from build123d import *

# Parameters (mm, degrees)
SKETCH_1_W          = 60
SKETCH_1_H          = 17
EXTRUDE_1_DEPTH     = 1.2
CUT_EXTRUDE_1_REACH = 33.204
SKETCH_4_R          = 3.25
SKETCH_4_W          = 9.6
SKETCH_4_H          = 3.4
SKETCH_4_W_2        = 7
SKETCH_4_H_2        = 3.5
SKETCH_4_W_3        = 8
SKETCH_4_H_3        = 2.9
SKETCH_4_W_4        = 8.4
SKETCH_4_H_4        = 3.2
SKETCH_4_W_5        = 6.5
FILLET_2_R          = 1
CHAMFER_1_SIZE      = 0.6
SKETCH_5_W          = 1.5
SKETCH_5_H          = 8
EXTRUDE_2_DEPTH     = 1.2
SKETCH_6_W          = 28.5
SKETCH_6_H          = 1.6
EXTRUDE_3_DEPTH     = 4
FILLET_3_R          = 1
CHAMFER_2_SIZE      = 1
CHAMFER_4_SIZE      = 1
FILLET_4_R          = 2
CHAMFER_5_SIZE      = 0.4


with BuildPart() as part:
    # 草图1 → 凸台-拉伸1 (new body)
    with BuildSketch(Plane(origin=(0, 0, 0), x_dir=(1, 0, 0), z_dir=(0, 1, 0))):
        Rectangle(SKETCH_1_W, SKETCH_1_H)
    extrude(amount=EXTRUDE_1_DEPTH)

    # 草图4 → 切除-拉伸1 (cut, up to next)
    with BuildSketch(Plane(origin=(0, 1.2, 0), x_dir=(1, 0, 0), z_dir=(0, 1, 0)), mode=Mode.PRIVATE) as cut_extrude_1_sk1:
        with Locations(Location((22.298485985, 3.98318929, 0), (0, 0, 270))):
            Circle(SKETCH_4_R)
    cut_extrude_1_tool1 = extrude(cut_extrude_1_sk1.sketch, amount=-CUT_EXTRUDE_1_REACH, mode=Mode.PRIVATE) & part.part
    # 草图4 → 切除-拉伸1 (cut, up to next)
    with BuildSketch(Plane(origin=(0, 1.2, 0), x_dir=(1, 0, 0), z_dir=(0, 1, 0)), mode=Mode.PRIVATE) as cut_extrude_1_sk2:
        with Locations((-20.471722325, 2.6)):
            Rectangle(SKETCH_4_W, SKETCH_4_H)
    cut_extrude_1_tool2 = extrude(cut_extrude_1_sk2.sketch, amount=-CUT_EXTRUDE_1_REACH, mode=Mode.PRIVATE) & part.part
    # 草图4 → 切除-拉伸1 (cut, up to next)
    with BuildSketch(Plane(origin=(0, 1.2, 0), x_dir=(1, 0, 0), z_dir=(0, 1, 0)), mode=Mode.PRIVATE) as cut_extrude_1_sk3:
        with Locations((-5.682926277, 2.55)):
            Rectangle(SKETCH_4_W_2, SKETCH_4_H_2)
    cut_extrude_1_tool3 = extrude(cut_extrude_1_sk3.sketch, amount=-CUT_EXTRUDE_1_REACH, mode=Mode.PRIVATE) & part.part
    # 草图4 → 切除-拉伸1 (cut, up to next)
    with BuildSketch(Plane(origin=(0, 1.2, 0), x_dir=(1, 0, 0), z_dir=(0, 1, 0)), mode=Mode.PRIVATE) as cut_extrude_1_sk4:
        with Locations((7.788485985, 2.55)):
            Rectangle(SKETCH_4_W_2, SKETCH_4_H_2)
    cut_extrude_1_tool4 = extrude(cut_extrude_1_sk4.sketch, amount=-CUT_EXTRUDE_1_REACH, mode=Mode.PRIVATE) & part.part
    # 草图4 → 切除-拉伸1 (cut, up to next)
    with BuildSketch(Plane(origin=(0, 1.2, 0), x_dir=(1, 0, 0), z_dir=(0, 1, 0)), mode=Mode.PRIVATE) as cut_extrude_1_sk5:
        with Locations((21.05, -4.584803861)):
            Rectangle(SKETCH_4_W_3, SKETCH_4_H_3)
    cut_extrude_1_tool5 = extrude(cut_extrude_1_sk5.sketch, amount=-CUT_EXTRUDE_1_REACH, mode=Mode.PRIVATE) & part.part
    # 草图4 → 切除-拉伸1 (cut, up to next)
    with BuildSketch(Plane(origin=(0, 1.2, 0), x_dir=(1, 0, 0), z_dir=(0, 1, 0)), mode=Mode.PRIVATE) as cut_extrude_1_sk6:
        with Locations((7.4, -4.734803861)):
            Rectangle(SKETCH_4_W_4, SKETCH_4_H_4)
    cut_extrude_1_tool6 = extrude(cut_extrude_1_sk6.sketch, amount=-CUT_EXTRUDE_1_REACH, mode=Mode.PRIVATE) & part.part
    # 草图4 → 切除-拉伸1 (cut, up to next)
    with BuildSketch(Plane(origin=(0, 1.2, 0), x_dir=(1, 0, 0), z_dir=(0, 1, 0)), mode=Mode.PRIVATE) as cut_extrude_1_sk7:
        with Locations((-7.25, -4.884803861)):
            Rectangle(SKETCH_4_W_5, SKETCH_4_H_2)
    cut_extrude_1_tool7 = extrude(cut_extrude_1_sk7.sketch, amount=-CUT_EXTRUDE_1_REACH, mode=Mode.PRIVATE) & part.part
    # 草图4 → 切除-拉伸1 (cut, up to next)
    with BuildSketch(Plane(origin=(0, 1.2, 0), x_dir=(1, 0, 0), z_dir=(0, 1, 0)), mode=Mode.PRIVATE) as cut_extrude_1_sk8:
        with Locations((-20.471722325, -4.834803861)):
            Rectangle(SKETCH_4_W, SKETCH_4_H)
    cut_extrude_1_tool8 = extrude(cut_extrude_1_sk8.sketch, amount=-CUT_EXTRUDE_1_REACH, mode=Mode.PRIVATE) & part.part
    add(cut_extrude_1_tool1.solids().sort_by_distance((22.298486, 1.2, -3.983189))[0], mode=Mode.SUBTRACT)
    add(cut_extrude_1_tool2.solids().sort_by_distance((-20.471722, 1.2, -2.6))[0], mode=Mode.SUBTRACT)
    add(cut_extrude_1_tool3.solids().sort_by_distance((-5.682926, 1.2, -2.55))[0], mode=Mode.SUBTRACT)
    add(cut_extrude_1_tool4.solids().sort_by_distance((7.788486, 1.2, -2.55))[0], mode=Mode.SUBTRACT)
    add(cut_extrude_1_tool5.solids().sort_by_distance((21.05, 1.2, 4.584804))[0], mode=Mode.SUBTRACT)
    add(cut_extrude_1_tool6.solids().sort_by_distance((7.4, 1.2, 4.734804))[0], mode=Mode.SUBTRACT)
    add(cut_extrude_1_tool7.solids().sort_by_distance((-7.25, 1.2, 4.884804))[0], mode=Mode.SUBTRACT)
    add(cut_extrude_1_tool8.solids().sort_by_distance((-20.471722, 1.2, 4.834804))[0], mode=Mode.SUBTRACT)

    # 圆角2
    fillet_2_edges = [part.edges().sort_by_distance(p)[0] for p in [
        (-9.182926277, 0.6, -4.3),
        (-2.182926277, 0.6, -4.3),
        (4.288485985, 0.6, -4.3),
        (11.288485985, 0.6, -4.3),
        (17.05, 0.6, 6.034803861),
        (25.05, 0.6, 6.034803861),
        (3.2, 0.6, 6.334803861),
        (3.2, 0.6, 3.134803861),
        (11.6, 0.6, 3.134803861),
        (11.6, 0.6, 6.334803861),
        (-10.5, 0.6, 6.634803861),
        (-10.5, 0.6, 3.134803861),
        (-4, 0.6, 3.134803861),
        (-4, 0.6, 6.634803861),
        (-25.271722325, 0.6, 6.534803861),
        (-25.271722325, 0.6, 3.134803861),
        (-15.671722325, 0.6, 3.134803861),
        (-15.671722325, 0.6, 6.534803861),
        (-25.271722325, 0.6, -0.9),
        (-25.271722325, 0.6, -4.3),
        (-15.671722325, 0.6, -4.3),
        (-15.671722325, 0.6, -0.9),
    ]]
    fillet(fillet_2_edges, radius=FILLET_2_R)

    # 倒角1
    chamfer_1_edges = [part.edges().sort_by_distance(p)[0] for p in [
        (-9.182926277, 0.6, -0.8),
        (-2.182926277, 0.6, -0.8),
        (4.288485985, 0.6, -0.8),
        (11.288485985, 0.6, -0.8),
        (17.05, 0.6, 3.134803861),
        (25.05, 0.6, 3.134803861),
    ]]
    chamfer(chamfer_1_edges, length=CHAMFER_1_SIZE)

    # 草图5 → 凸台-拉伸2 (add)
    with BuildSketch(Plane.XZ):
        with Locations((-13.15891381, 0.61681071)):
            Rectangle(SKETCH_5_W, SKETCH_5_H)
        with Locations((13.84108619, 0.61681071)):
            Rectangle(SKETCH_5_W, SKETCH_5_H)
    extrude(amount=EXTRUDE_2_DEPTH)

    # 草图6 → 凸台-拉伸3 (add)
    with BuildSketch(Plane.XZ):
        with Locations((0.34108619, 1.3)):
            Rectangle(SKETCH_6_W, SKETCH_6_H)
    extrude(amount=EXTRUDE_3_DEPTH)

    # 圆角3
    fillet_3_edges = [part.edges().sort_by_distance(p)[0] for p in [
        (-13.90891381, -4, 1.3),
        (14.59108619, -4, 1.3),
    ]]
    fillet(fillet_3_edges, radius=FILLET_3_R)

    # 倒角2
    chamfer_2_edges = [part.edges().sort_by_distance(p)[0] for p in [
        (-13.15891381, -1.2, -3.38318929),
        (-13.15891381, -1.2, 4.61681071),
        (13.84108619, -1.2, -3.38318929),
        (13.84108619, -1.2, 4.61681071),
    ]]
    chamfer(chamfer_2_edges, length=CHAMFER_2_SIZE)

    # 倒角4
    chamfer_4_edges = [part.edges().sort_by_distance(p)[0] for p in [
        (-5.682926277, 0, -4.3),
        (-2.182926277, 0, -2.35),
        (7.788485985, 0, -4.3),
        (11.288485985, 0, -2.35),
        (21.05, 0, 6.034803861),
        (17.05, 0, 4.384803861),
        (-2.475819496, 0, -4.007106781),
        (-8.890033058, 0, -4.007106781),
        (4.581379204, 0, -4.007106781),
        (10.995592766, 0, -4.007106781),
        (24.757106781, 0, 5.741910642),
        (17.342893219, 0, 5.741910642),
        (-5.682926277, 0, -0.8),
        (-9.182926277, 0, -2.35),
        (7.788485985, 0, -0.8),
        (4.288485985, 0, -2.35),
        (21.05, 0, 3.134803861),
        (25.05, 0, 4.384803861),
        (-8.882926277, 0, -1.1),
        (-2.482926277, 0, -1.1),
        (4.588485985, 0, -1.1),
        (10.988485985, 0, -1.1),
        (17.35, 0, 3.434803861),
        (24.75, 0, 3.434803861),
    ]]
    chamfer(chamfer_4_edges, length=CHAMFER_4_SIZE)

    # 圆角4
    fillet_4_edges = [part.edges().sort_by_distance(p)[0] for p in [
        (30, 0.6, 8.5),
        (-30, 0.6, 8.5),
        (-30, 0.6, -8.5),
        (30, 0.6, -8.5),
    ]]
    fillet(fillet_4_edges, radius=FILLET_4_R)

    # 倒角5
    chamfer_5_edges = [part.edges().sort_by_distance(p)[0] for p in [
        (30, 0, 0),
        (0, 0, 8.5),
        (-30, 0, 0),
        (0, 0, -8.5),
        (-29.414213562, 0, -7.914213562),
        (-29.414213562, 0, 7.914213562),
        (29.414213562, 0, -7.914213562),
        (29.414213562, 0, 7.914213562),
    ]]
    chamfer(chamfer_5_edges, length=CHAMFER_5_SIZE)


solid = part.part
The model under review builds one solid part; all positions refer to its coordinate system, in mm. A direction names the side the tool comes from. Give positions to 0.01 mm unless a question says otherwise; leave off trailing zeros. Order: outer loops, then holes, each group sorted by start corner. A loop starts at its lowest first (then second) coordinate and runs counter-clockwise, first axis right, second up. Notation, with made-up numbers: M -26.75,30 L -22.75,30 A23 ccw -22.75,62 Z; hole C 3,62 d11. An arc over 180 degrees is marked long. Use one line per item in the form item = value. Start each with the question number.
Item 1: Insertion check: pin 1 Ø2 at (y, z) = (-2, -5.5) entering from +X; pin 2 Ø4 at (x, z) = (-5.5, -3.5) entering from -Y; pin 3 Ø1 at (y, z) = (-1, -1.5) entering from -X; pin 4 Ø1.5 at (x, y) = (15, -2.5) entering from +Z. Each pin has a flat end and moves straight along its axis. Give the tip position at first contact, or say it passes through.
Item 2: For faces 1 (the flat face through (13.091, -1, -1)), 2 (the flat face through (-25.272, 1, -3)), 3 (the flat face through (3.8, 0.51, -2.16)), 4 (the flat face through (13.091, -1, 3)), 5 (the conical face through (29.225, 0.114, -7.699)), list the 3-axis set-ups (+Z, -Z, +X, -X, +Y, -Y) from which the entire face can be reached by the end or side of a thin tool; tool diameter is ignored.
Item 3: We need section A-A on x = 9. Give the boundary of the cut face in (y, z), plus the area to 3 significant figures.
Item 4: The part is to be moulded in two halves that separate along X. For faces 6 (the cylindrical face through (-29.43, 0.81, -7.9)), 7 (the cylindrical face through (-24.987, 0.592, -3.999)), 8 (the cylindrical face through (29.4, 0.81, 7.93)), say which applies: pulls with the +X half, pulls with the -X half, needs draft (parallel to the pull), parting line crosses it, or undercut.
Item 5: To check wall thickness, follow line 1 along X through (y, z) = (0.3, -4); line 2 along X through (y, z) = (-0.75, -2.5); line 3 along Y through (x, z) = (4, -6.75). State the ranges of each line that lie inside material, in increasing order. Write a range as from..to.
Completed:
q1.pin_1 = through
q1.pin_2 = 0
q1.pin_3 = -13.91
q1.pin_4 = 2.1
q2.face_1 = -Z, -Y
q2.face_2 = +Y, -Y
q2.face_3 = -Y
q2.face_4 = +Z, -Y
q2.face_5 = -Z, +X, -Y
q3.outline = M -4,0.5 L 0,0.5 L 0,0.2 L 1,-0.8 L 1.2,-0.8 L 1.2,3.13 L 0,3.13 L 0,2.1 L -4,2.1 Z; M 0,-8.1 L 0.4,-8.5 L 1.2,-8.5 L 1.2,-4.3 L 1,-4.3 L 0,-5.3 Z; M 0,6.33 L 1.2,6.33 L 1.2,8.5 L 0.4,8.5 L 0,8.1 Z
q3.area = 17.6 mm²
q4.face_6 = pulls with the -X half
q4.face_7 = undercut
q4.face_8 = pulls with the +X half
q5.line_1 = -29.9..-24.99, -15.96..-9.73, -1.63..3.74, 11.84..19.05, 25.55..29.9
q5.line_2 = -13.91..-12.41, 13.09..14.59
q5.line_3 = 0..1.2
